CAD build for the part. Positions are in the model's coordinates, mm. A direction names the side the tool comes from. Coordinates: 2 decimals unless noted, no trailing zeros. Loops run counter-clockwise (first coordinate to the right, second up) from the corner with the lowest first, then second, coordinate; pieces in that order, holes last. Notation, with made-up numbers: M 44.25,7.25 L 93.25,7.25 A20 ccw 93.25,45.25 Z; hole C -6,80.25 d5. An arc over 180 degrees is marked long. Answer as a JSON object with one key per item and string values. Group by question number.
```python
from build123d import *

# Parameters (mm, degrees)
SKETCH1_R           = 214.63
SKETCH1_R_2         = 25.4
BOSS_EXTRUDE1_DEPTH = 6.35
SKETCH3_R           = 3.2893
CUT_EXTRUDE2_DEPTH  = 7.35
CUT_EXTRUDE3_DEPTH  = 7.35


with BuildPart() as part:
    # Sketch1 → Boss-Extrude1 (new body)
    with BuildSketch(Plane(origin=(0, 0, 0), x_dir=(1, 0, 0), z_dir=(0, 1, 0))):
        Circle(SKETCH1_R)
        Circle(SKETCH1_R_2, mode=Mode.SUBTRACT)
    extrude(amount=BOSS_EXTRUDE1_DEPTH)

    # Sketch3 → Cut-Extrude2 (cut, through all)
    with BuildSketch(Plane(origin=(0, 6.35, 0), x_dir=(1, 0, 0), z_dir=(0, 1, 0))):
        with Locations((0, 31.75)):
            Circle(SKETCH3_R)
        with Locations((31.75, 0)):
            Circle(SKETCH3_R)
        with Locations((0, -31.75)):
            Circle(SKETCH3_R)
        with Locations((-31.75, 0)):
            Circle(SKETCH3_R)
    extrude(amount=-CUT_EXTRUDE2_DEPTH, mode=Mode.SUBTRACT)

    # Sketch4 → Cut-Extrude3 (cut, through all)
    with BuildSketch(Plane(origin=(0, 6.35, 0), x_dir=(1, 0, 0), z_dir=(0, 1, 0))):
        with BuildLine():
            Line((25.4, 170.18), (25.4, 69.85))
            ThreePointArc((25.4, 69.85), (0, 44.45), (-25.4, 69.85))
            Line((-25.4, 69.85), (-25.4, 170.18))
            ThreePointArc((-25.4, 170.18), (0, 195.58), (25.4, 170.18))
        make_face()
        with BuildLine():
            Line((170.18, -25.4), (69.85, -25.4))
            ThreePointArc((69.85, -25.4), (44.45, 0), (69.85, 25.4))
            Line((69.85, 25.4), (170.18, 25.4))
            ThreePointArc((170.18, 25.4), (195.58, 0), (170.18, -25.4))
        make_face()
        with BuildLine():
            Line((-25.4, -170.18), (-25.4, -69.85))
            ThreePointArc((-25.4, -69.85), (0, -44.45), (25.4, -69.85))
            Line((25.4, -69.85), (25.4, -170.18))
            ThreePointArc((25.4, -170.18), (0, -195.58), (-25.4, -170.18))
        make_face()
        with BuildLine():
            Line((-170.18, 25.4), (-69.85, 25.4))
            ThreePointArc((-69.85, 25.4), (-44.45, 0), (-69.85, -25.4))
            Line((-69.85, -25.4), (-170.18, -25.4))
            ThreePointArc((-170.18, -25.4), (-195.58, 0), (-170.18, 25.4))
        make_face()
    extrude(amount=-CUT_EXTRUDE3_DEPTH, mode=Mode.SUBTRACT)


solid = part.part
```
Item 1: Slice it at A-A, the plane z = -90. Write the cut outline in (x, y).
Item 2: Slice it at D-D, the plane z = 10. Write the cut outline in (x, y).
Item 3: Pull direction X, two halves, no side cores. Call faces 3 (the cylindrical face through (-5.506, 3.131, 24.796)), 4 (the flat face through (45, 6.35, 45)), 5 (the cylindrical face through (115.38, 3.13, -180.98)): released by +X, released by -X, zero draft, split by the parting line, or undercut.
Item 4: Slice it at B-B, the plane y = 1.5. Count the separate pieces of the cut face and the enclosed holes in it, then the cut area to 3 significant figures.
Item 5: Drill centre lines: L1, parallel to X at y = 2.5, z = 0; L2, parallel to Z at x = 7.5, y = 2.25. Where is each one in solid material? Low to high. Write a range as from..to.
Item 6: Slice it at C-C, the plane x = -155.5. Write the cut outline in (y, z), then the cut area to 3 significant figures.
Item 7: Tool access for faces 1 (the cylindrical face through (-0.559, 3.219, 44.456)), 2 (the flat face through (45, 0, 45)): list every direction of +Z, -Z, +X, -X, +Y, -Y with a clear straight run to the whole face (end or side of a thin tool).
Item 8: Pin check, flat tips, straight feed: pin 1 (1.9 mm diameter, centred on x = -105.5, y = 3.5, fed in from +Z); pin 2 (3 mm diameter, centred on y = 4.5, z = -128, fed in from +X); pin 3 (3 mm diameter, centred on x = -38, y = 3, fed in from -Z). Stop position of each tip, or through.
Computed:
{
 "1": {"outline": "M -194.85,0 L -25.4,0 L -25.4,6.35 L -194.85,6.35 Z; M 25.4,0 L 194.85,0 L 194.85,6.35 L 25.4,6.35 Z"},
 "2": {"outline": "M -214.4,0 L -193.53,0 L -193.53,6.35 L -214.4,6.35 Z; M -46.5,0 L -23.35,0 L -23.35,6.35 L -46.5,6.35 Z; M 23.35,0 L 46.5,0 L 46.5,6.35 L 23.35,6.35 Z; M 193.53,0 L 214.4,0 L 214.4,6.35 L 193.53,6.35 Z"},
 "3": {"face 3": "undercut", "face 4": "zero draft", "face 5": "split by the parting line"},
 "4": {"separate pieces": "1", "enclosed holes": "9", "area": "114,000 mm2"},
 "5": {"L1": "-214.63..-195.58, -44.45..-35.04, -28.46..-25.4, 25.4..28.46, 35.04..44.45, 195.58..214.63", "L2": "-214.5..-194.45, -45.58..-24.27, 24.27..45.58, 194.45..214.5"},
 "6": {"outline": "M 0,-147.94 L 6.35,-147.94 L 6.35,-25.4 L 0,-25.4 Z; M 0,25.4 L 6.35,25.4 L 6.35,147.94 L 0,147.94 Z", "area": "1,560 mm2"},
 "7": {"face 1": "+Y, -Y", "face 2": "+Z, -Z, +X, -X, -Y"},
 "8": {"pin 1": "z = 187.44", "pin 2": "x = 173.39", "pin 3": "z = -211.5"}
}
